Design review of the part shown in the three views and the two pictorial views. Dimensions are in mm from the part's minimum x, y and z. A direction names the side the tool comes from. Coordinates: 2 decimals unless noted, no trailing zeros. Write each loop counter-clockwise with the first axis right and the second up, starting at its lowest first coordinate (ties: lowest second). Pieces come first, ordered by that corner, then holes. Notation, with made-up numbers: (-26, 18) - (28, 18) arc R32 ccw to (28, 49) - close; hole circle Ø3 at (4, 69). An arc over 180 degrees is marked (long way). Return JSON: item names as keys, results as strings. Group by question number.
(1) We need section D-D on x = 2. State the section outline as (y, z) points, then the cut area to 3 significant figures.
(2) To check wall thickness, follow L1, parallel to Y at x = 6.5, z = 34; L2, parallel to Z at x = 8.25, y = 9.25; L3, parallel to X at y = 4.5, z = 33.5. State the ranges of each line that lie inside material, in increasing order. Write a range as from..to.
(3) Tool access review of the marked faces 1, 2 and 3: name each direction out of +Z, -Z, +X, -X, +Y, -Y from which nothing blocks a thin tool from reaching the whole face with its end or side.
(4) We need section C-C on x = 6. State the section outline as (y, z) points, then the cut area to 3 significant figures.
(5) We need section A-A on y = 6. State the section outline as (x, z) points.
(6) For pin 1 Ø2 at (y, z) = (6.5, 34) entering from +X; pin 2 Ø4.5 at (y, z) = (6, 33.5) entering from -X; pin 3 Ø5 at (y, z) = (2.5, 12) entering from +X, all flat-tipped, find the tip position at first contact; note any pin that passes through.
(7) We need section B-B on z = 34. State the section outline as (x, y) points.
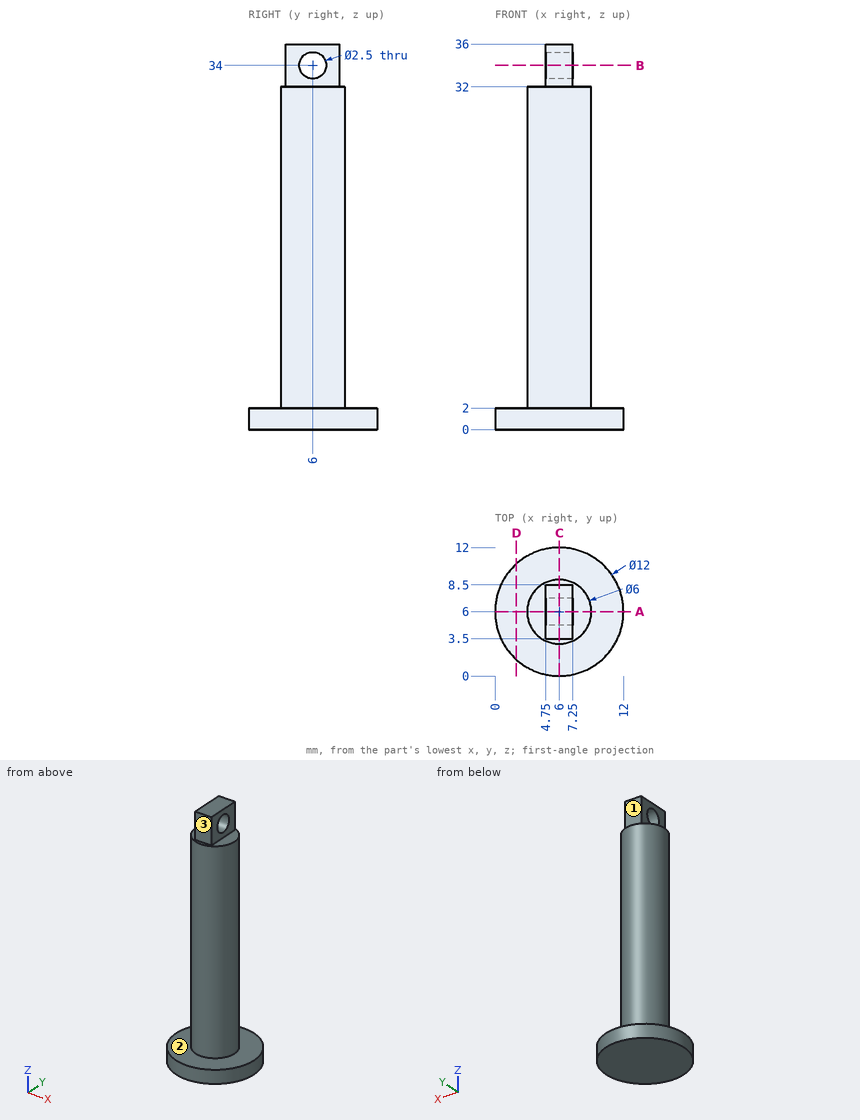
Ans:
{
 "1": {"outline": "(1.53, 0) - (10.47, 0) - (10.47, 2) - (1.53, 2) - close", "area": "17.9 mm²"},
 "2": {"L1": "3.5..4.75, 7.25..8.5", "L2": "0..2", "L3": "4.75..7.25"},
 "3": {"face 1": "+Z, +X, -X, +Y", "face 2": "+Z", "face 3": "+Z, +X, -X, -Y"},
 "4": {"outline": "(0, 0) - (12, 0) - (12, 2) - (9, 2) - (9, 32) - (8.5, 32) - (8.5, 36) - (3.5, 36) - (3.5, 32) - (3, 32) - (3, 2) - (0, 2) - close; hole circle Ø2.5 at (6, 34)", "area": "219 mm²"},
 "5": {"outline": "(0, 0) - (12, 0) - (12, 2) - (9, 2) - (9, 32) - (7.25, 32) - (7.25, 32.75) - (4.75, 32.75) - (4.75, 32) - (3, 32) - (3, 2) - (0, 2) - close; (4.75, 35.25) - (7.25, 35.25) - (7.25, 36) - (4.75, 36) - close"},
 "6": {"pin 1": "x = 7.25", "pin 2": "x = 3", "pin 3": "x = 8.83"},
 "7": {"outline": "(4.75, 3.5) - (7.25, 3.5) - (7.25, 4.75) - (4.75, 4.75) - close; (4.75, 7.25) - (7.25, 7.25) - (7.25, 8.5) - (4.75, 8.5) - close"}
}
